from build123d import *

# Parameters (mm, degrees)
BASE_START       = -160
SKETCH_6_W       = 200
SKETCH_6_H       = 100
BASE_PLATE_DEPTH = 10
POST_START       = 150
SKETCH_7_R       = 25
POST_DEPTH       = 300
TOP_START        = 150
SKETCH_8_W       = 200
SKETCH_8_H       = 60
TOP_PLATE_DEPTH  = 11.5


with BuildPart() as part:
    # 草图6 → Base Plate (new body)
    with BuildSketch(Plane(origin=(0, 0, 0), x_dir=(1, 0, 0), z_dir=(0, 1, 0)).offset(BASE_START)):
        Rectangle(SKETCH_6_W, SKETCH_6_H)
    extrude(amount=BASE_PLATE_DEPTH)

    # 草图7 → Post (add)
    with BuildSketch(Plane(origin=(0, 0, 0), x_dir=(1, 0, 0), z_dir=(0, 1, 0)).offset(POST_START)):
        with Locations(Location((0, 0, 0), (0, 0, 270))):
            Circle(SKETCH_7_R)
    extrude(amount=-POST_DEPTH)

    # 草图8 → Top Plate (add)
    with BuildSketch(Plane(origin=(0, 0, 0), x_dir=(1, 0, 0), z_dir=(0, 1, 0)).offset(TOP_START)):
        Rectangle(SKETCH_8_W, SKETCH_8_H)
    extrude(amount=TOP_PLATE_DEPTH)


solid = part.part
Part model, mm, in its own coordinate system. A direction names the side the tool comes from. Coordinates: 2 decimals unless noted, no trailing zeros. Write each loop counter-clockwise with the first axis right and the second up, starting at its lowest first coordinate (ties: lowest second). Pieces come first, ordered by that corner, then holes. Notation, with made-up numbers: M 64,48 L 94,48 A24 ccw 94,75 Z; hole C 29,-6 d5. An arc over 180 degrees is marked long. Return JSON: item names as keys, results as strings.
1. Flat gauge pins, fed straight in: pin 1 Ø3.5 at (x, y) = (-41, 155) entering from +Z; pin 2 Ø3.5 at (x, y) = (-49, 158.5) entering from -Z; pin 3 Ø10 at (y, z) = (-5.5, 2.5) entering from +X. Where does each tip first touch, or does it go through?
Determined:
{"pin 1": "z = 30", "pin 2": "z = -30", "pin 3": "x = 25"}
2. Saw through at B-B, the plane z = 0. Write the cut outline in (x, y), then the cut area to 3 significant figures.
Determined:
{"outline": "M -100,-160 L 100,-160 L 100,-150 L 25,-150 L 25,150 L 100,150 L 100,161.5 L -100,161.5 L -100,150 L -25,150 L -25,-150 L -100,-150 Z", "area": "19,300 mm²"}
3. Pull direction Y, two halves, no side cores. Call faces 4 (the face through (-1, 161.5, 0)), 5 (the face through (7.509, 2.1, 23.846)), 6 (the face through (-24, 150, -14)), 7 (the face through (-1, 156, -30)): pulls with the +Y half, pulls with the -Y half, needs draft (parallel to the pull), parting line crosses it, or undercut.
Determined:
{"face 4": "pulls with the +Y half", "face 5": "undercut", "face 6": "undercut", "face 7": "needs draft"}
4. Saw through at A-A, the plane x = -79.5. Write the cut outline in (y, z).
Determined:
{"outline": "M -160,-50 L -150,-50 L -150,50 L -160,50 Z; M 150,-30 L 161.5,-30 L 161.5,30 L 150,30 Z"}
5. Probe L1, parallel to Y at x = -28.5, z = 22.5; L2, parallel to Y at x = -14, z = 35; L3, parallel to X at y = -102.5, z = 18. List the from-to ranges inside material, lowest first.
Determined:
{"L1": "-160 to -150, 150 to 161.5", "L2": "-160 to -150", "L3": "-17.35 to 17.35"}
6. Saw through at D-D, the plane y = 55.5. Write the cut outline in (x, z), then the cut area to 3 significant figures.
Determined:
{"outline": "C 0,0 d50", "area": "1,960 mm²"}
7. Saw through at C-C, the plane x = 0. Write the cut outline in (y, z), then the cut area to 3 significant figures.
Determined:
{"outline": "M -160,-50 L -150,-50 L -150,-25 L 150,-25 L 150,-30 L 161.5,-30 L 161.5,30 L 150,30 L 150,25 L -150,25 L -150,50 L -160,50 Z", "area": "16,700 mm²"}
8. 3-axis set-ups, long thin cutter, end or side, ignore diameter. For faces 1 (the face through (-1, 156, 30)), 2 (the face through (-24, -150, -12)), 3 (the face through (-1, -155, 50)): which of +Z, -Z, +X, -X, +Y, -Y reach the whole face in a straight line?
Determined:
{"face 1": "+Z, +X, -X, +Y", "face 2": "none", "face 3": "+Z, +X, -X, +Y, -Y"}
